Autodesk Inventor part; units mm, degrees
ref_plane "YZ Plane" through (0, 0, 0) normal (1, 0, 0) x (0, 1, 0)
ref_plane "XZ Plane" through (0, 0, 0) normal (0, 1, 0) x (-1, 0, 0)
ref_plane "XY Plane" through (0, 0, 0) normal (0, 0, 1) x (1, 0, 0)
sketch "Sketch1" plane through (0, 0, 0) normal (0, 0, 1) x (1, 0, 0)
  arc A0 (-87.5, 200) -> (87.5, 200) centre (0, 200) ccw
  line L0 (87.5, 200) -> (125, 200)
  line L1 (125, 200) -> (125, 0)
  line L2 (125, 0) -> (-107, 0)
  line L3 (-107, 0) -> (-107, 200)
  line L4 (-107, 200) -> (-87.5, 200)
  point P0 (0, 0)
  dimension "d0" = 200
  dimension "d1" = 175
  dimension "d2" = 37.5
  dimension "d3" = 232
  dimension "d4" = 125
  dimension "d5" = 200
extrude "Extrusion1" add sketch "Sketch1" against normal blind 20
properties part number "Weldedsupportpart1"
CAD build for the part. Positions are in the model's coordinates, mm. Give positions to 0.01 mm unless a question says otherwise; leave off trailing zeros. Order: outer loops, then holes, each group sorted by start corner. A loop starts at its lowest first (then second) coordinate and runs counter-clockwise, first axis right, second up. Notation, with made-up numbers: M -13,-6.5 L 12,-6.5 A14 cw 12,3.5 Z; hole C -30.75,50 d10. An arc over 180 degrees is marked long. Put each result on its own line as item: value. Start each with the question number.
(1) Saw through at C-C, the plane x = -80. Write the cut outline in (y, z), then the cut area to 3 significant figures.
(2) Saw through at A-A, the plane z = -7. Write the cut outline in (x, y).
(3) Drill centre lines: line 1 along X through (y, z) = (174, -16); line 2 along X through (y, z) = (167, -9.5); line 3 along Y through (x, z) = (-62, -2.75). Where is each one in solid material? Low to high.
(4) Flat gauge pins, fed straight in: pin 1 Ø4 at (x, z) = (1.5, -11.5) entering from +Y; pin 2 Ø1.5 at (x, z) = (-6.5, -16.5) entering from +Y; pin 3 Ø8 at (x, z) = (-20, -11) entering from +Y. Where does each tip first touch, or does it go through?
(5) Saw through at B-B, the plane x = 0. Write the cut outline in (y, z).
Check result:
1. outline: M 0,-20 L 164.56,-20 L 164.56,0 L 0,0 Z
1. area: 3,290 mm2
2. outline: M -107,0 L 125,0 L 125,200 L 87.5,200 A87.5 cw -87.5,200 L -107,200 Z
3. line 1: x = -107 to -83.55, 83.55 to 125
3. line 2: x = -107 to -81.04, 81.04 to 125
3. line 3: y = 0 to 138.26
4. pin 1: stops at y = 112.57
4. pin 2: stops at y = 112.8
4. pin 3: stops at y = 115.86
5. outline: M 0,-20 L 112.5,-20 L 112.5,0 L 0,0 Z
